The model under review builds one solid part; all positions refer to its coordinate system, in mm. Face numbers are marked on the shaded views. Give positions to 0.01 mm unless a question says otherwise; leave off trailing zeros. Loops run counter-clockwise (first coordinate to the right, second up) from the corner with the lowest first, then second, coordinate; pieces in that order, holes last. Notation, with made-up numbers: M 1.25,76 L 53.25,76 A18 ccw 53.25,97 Z; hole C 50,15.25 d4. An arc over 180 degrees is marked long. One line per item, written item: value. Start each with the question number.
Q1. We need section A-A on x = 6. Write out the cut boundary in (y, z), plus the area to 3 significant figures.
Q2. We need section C-C on x = -20.5. Write out the cut boundary in (y, z), plus the area to 3 significant figures.
Q3. We need section D-D on y = 2.5. Write out the cut boundary in (x, z), plus the area to 3 significant figures.
Q4. For pin 1 (1 mm diameter, centred on x = -15.5, y = -23.5, fed in from +Z), flat-tipped, find the tip position at first contact; note if it passes through.
Q5. Mouldability with a two-part tool opening along Y and no side actions: class the marked faces 1, 2 and 3 as released by +Y, released by -Y, zero draft, split by the parting line, or undercut.
Q6. To check wall thickness, follow line 1 along X through (y, z) = (-22.5, 15); line 2 along Y through (x, z) = (6, 12.5); line 3 along Z through (x, y) = (-19, 11.5). State the ranges of each line that lie inside material, in increasing order. Write a range as from..to.
```python
from build123d import *

# Parameters (mm, degrees)
F0_W        = 215.5817523599
F0_H        = 32.4833281338
F1_DEPTH    = 25.908
F2_T1_DEPTH = 1087.9500123763
F4_DEPTH    = 9.398


# Not quite as in the source:
# - a fillet or chamfer that OpenCascade refuses, or shapes differently, is made with other operations: its cross-section is extruded or revolved along the edge and cut away or added


with BuildPart() as f1:
    # F0 (on Right) → F1 (new body)
    with BuildSketch(Plane.YZ):
        with Locations((-13.4214349091, 16.2416640669)):
            Rectangle(F0_W, F0_H)
    extrude(amount=-F1_DEPTH)

    # F2: fillet of radius 710.7106737728 on 1 edges, made by hand

    # F2_s2 → F2_t1 (cut)
    with BuildSketch(Plane.YZ.offset(-556.9290061881)):
        with BuildLine():
            ThreePointArc((91.1960913862, 32.4833281338), (-16.2428401618, 24.3155625185), (-121.212311089, 0))
            Line((-121.212311089, 0), (-121.212311089, 32.4833281338))
            Line((-121.212311089, 32.4833281338), (91.1960913862, 32.4833281338))
        make_face()
    extrude(amount=F2_T1_DEPTH, mode=Mode.SUBTRACT)

    # F3 (on face) → F4 (join)
    with BuildSketch(Plane.YZ):
        with BuildLine():
            ThreePointArc((-41.9370249708, 0), (-39.3490534124, 3.0127715747), (-38.4182262134, 6.873853039))
            ThreePointArc((-38.4182262134, 6.873853039), (-50.7526254785, 14.4163436408), (-51.8460630576, 0))
            Line((-51.8460630576, 0), (-41.9370249708, 0))
        make_face()
        with BuildLine():
            ThreePointArc((80.2152858595, 9.5448940992), (59.8493914636, 23.9956386528), (52.9354202211, 0))
            Line((52.9354202211, 0), (76.8756431877, 0))
            ThreePointArc((76.8756431877, 0), (79.356276258, 4.4887538584), (80.2152858595, 9.5448940992))
        make_face()
    extrude(amount=F4_DEPTH)


solid = f1.part
```
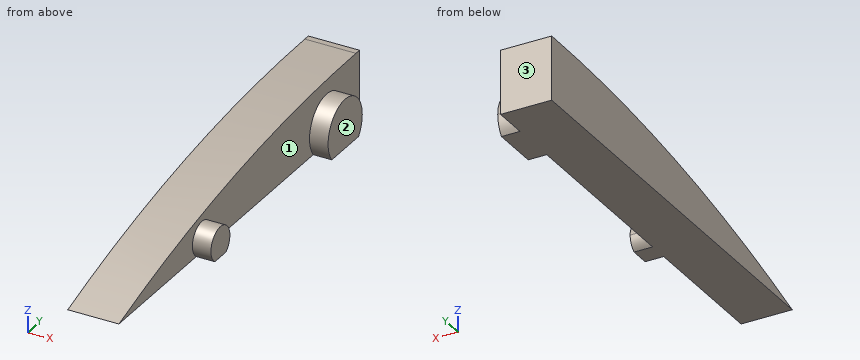
Solved:
1. outline: M -51.85,0 L -41.94,0 A8.47 ccw long Z; M 52.94,0 L 76.88,0 A15.31 ccw long Z
1. area: 855 mm2
2. outline: M -121.21,0 L 94.37,0 L 94.37,32.48 L 91.2,32.48 A710.71 ccw Z
2. area: 4,720 mm2
3. outline: M -25.91,0 L 0,0 L 0,26.93 L -25.91,26.93 Z
3. area: 698 mm2
4. pin 1: z = 23.25
5. face 1: undercut
5. face 2: zero draft
5. face 3: released by +Y
6. line 1: -25.91..0
6. line 2: -53.23..-40.56, 49.88..79.93
6. line 3: 0..28
